Model file for the job. Use its own axes, mm. Give positions to 0.01 mm unless a question says otherwise; leave off trailing zeros. Write each loop counter-clockwise with the first axis right and the second up, starting at its lowest first coordinate (ties: lowest second). Pieces come first, ordered by that corner, then holes. Notation, with made-up numbers: (89.5, -20.5) - (114.5, -20.5) arc R30 cw to (114.5, 11.5) - close; hole circle Ø11 at (15, 72.25). An arc over 180 degrees is marked (long way). Use CSV: the item, a comma, the result in double quotes.
from build123d import *

# Parameters (mm, degrees)
PAD004_DEPTH         = 25
FILLET005_R          = 2
SKETCH009_R          = 2
POCKET004_DEPTH      = 11.420051
POCKET004_DEPTH_BACK = 11.420051


with BuildPart() as part:
    # Sketch008 → Pad004 (new body)
    with BuildSketch(Plane.XY):
        with BuildLine():
            ThreePointArc((-7.239723, 11.419051), (-10, 0), (-7.239723, -11.419051))
            Line((-18.540393, -8), (-7.239723, -11.419051))
            Line((-35, -8), (-18.540393, -8))
            Line((-35, 8), (-35, -8))
            Line((-18.540393, 8), (-35, 8))
            Line((-7.239723, 11.419051), (-18.540393, 8))
        make_face()
    extrude(amount=PAD004_DEPTH)

    # Fillet005
    fillet005_edges = [part.edges().sort_by_distance(p)[0] for p in [
        (-35, 0, 25),
        (-35, 0, 0),
    ]]
    fillet(fillet005_edges, radius=FILLET005_R)

    # Sketch009 → Pocket004 (cut, two sides)
    with BuildSketch(Plane.XZ) as pocket004_sk:
        with Locations((-27, 12.5)):
            Circle(SKETCH009_R)
    extrude(amount=-POCKET004_DEPTH, mode=Mode.SUBTRACT)
    extrude(pocket004_sk.sketch, amount=POCKET004_DEPTH_BACK, mode=Mode.SUBTRACT)


with BuildPart() as part_1:
    # Body004 placement: moved
    add(part.part.moved(Location((90, 0, 0))))


solid = part_1.part
(1) Saw through at A-A, the plane x = 63. List the corners of the cut face in (y, z).
Checked values:
outline,"(-8, 0) - (8, 0) - (8, 10.5) - (-8, 10.5) - close; (-8, 14.5) - (8, 14.5) - (8, 25) - (-8, 25) - close"
(2) Pull direction Y, two halves, no side cores. Call faces 1 (the face through (65.2, 8, 12.3)), 2 (the face through (63, -8, 10)), 3 (the face through (80, 0, 12)), 4 (the face through (55, 0, 12)): released by +Y, released by -Y, zero draft, split by the parting line, or undercut.
Checked values:
face 1,"released by +Y"
face 2,"released by -Y"
face 3,"undercut"
face 4,"zero draft"
(3) Saw through at D-D, the plane z = 16.25. List the corners of the cut face in (x, y).
Checked values:
outline,"(55, -8) - (71.46, -8) - (82.76, -11.42) arc R25 cw to (82.76, 11.42) - (71.46, 8) - (55, 8) - close"
(4) Wall check: probe 1 along Z at (x, y) = (63, 3); probe 2 along Y at (x, z) = (62.75, 15); probe 3 along X at (y, z) = (-0.75, 10.75). Give the ranges that are in metal, low to high. Write a range as [from, to].
Checked values:
probe 1,"z = [0, 10.5], [14.5, 25]"
probe 2,"y = [-8, 8]"
probe 3,"x = [55, 62.03], [63.97, 80.01]"
(5) Flat gauge pins, fed straight in: P1, Ø3, axis at x = 64.5, z = 12, coming from the -Y side; P2, Ø13, axis at x = 66.5, z = 7.5, coming from the -Y side; P3, Ø1.5, axis at x = 65, z = 7, coming from the +Y side. Where does each tip first touch, or does it go through?
Checked values:
P1,"stops at y = -8"
P2,"stops at y = -8.47"
P3,"stops at y = 8"
(6) Saw through at B-B, the plane z = 12.5. List the corners of the cut face in (x, y), then the cut area to 3 significant figures.
Checked values:
outline,"(55, -8) - (61, -8) - (61, 8) - (55, 8) - close; (65, -8) - (71.46, -8) - (82.76, -11.42) arc R25 cw to (82.76, 11.42) - (71.46, 8) - (65, 8) - close"
area,"376 mm^2"
(7) Saw through at C-C, the plane y = -4.5. List the corners of the cut face in (x, z).
Checked values:
outline,"(55, 2) arc R2 ccw to (57, 0) - (80.41, 0) - (80.41, 25) - (57, 25) arc R2 ccw to (55, 23) - close; hole circle Ø4 at (63, 12.5)"
